Input: part model. Units: mm. Frame: model coordinates. Face numbers are marked on the shaded views. Give positions to 0.01 mm unless a question says otherwise; leave off trailing zeros. Write each loop counter-clockwise with the first axis right and the second up, starting at its lowest first coordinate (ties: lowest second). Pieces come first, ordered by that corner, then holes. Notation, with made-up numbers: (66.25, -18.5) - (122.25, -18.5) arc R16 ccw to (122.25, -9.5) - close; hole circle Ø5 at (42, 54.25). An arc over 180 degrees is marked (long way). Answer as CSV lines item,"result".
```python
from build123d import *

# Parameters (mm, degrees)
SKETCH1_R           = 7.5
BOSS_EXTRUDE1_DEPTH = 10
SKETCH2_R           = 6.5
CUT_EXTRUDE1_DEPTH  = 8.5
CAVITY1_START       = 8
CAVITY1_OUTLINE_R   = 6.6
CAVITY1_DEPTH       = 0.5


# Read off the part's stored shape, not the designer's step: Cavity1
with BuildPart() as part:
    # Sketch1 → Boss-Extrude1 (new body)
    with BuildSketch(Plane(origin=(0, 0, 0), x_dir=(1, 0, 0), z_dir=(0, 1, 0))):
        with Locations(Location((0, 0, 0), (0, 0, 270))):
            Circle(SKETCH1_R)
    extrude(amount=BOSS_EXTRUDE1_DEPTH)

    # Sketch2 → Cut-Extrude1 (cut)
    with BuildSketch(Plane(origin=(0, 10, 0), x_dir=(1, 0, 0), z_dir=(0, 1, 0))):
        with Locations(Location((0, 0, 0), (0, 0, 270))):
            Circle(SKETCH2_R)
    extrude(amount=-CUT_EXTRUDE1_DEPTH, mode=Mode.SUBTRACT)

    # Cavity1 outline → Cavity1 (cut)
    with BuildSketch(Plane(origin=(0, 0, 0), x_dir=(1, 0, 0), z_dir=(0, 1, 0)).offset(CAVITY1_START)):
        Circle(CAVITY1_OUTLINE_R)
    extrude(amount=CAVITY1_DEPTH, mode=Mode.SUBTRACT)


solid = part.part
```
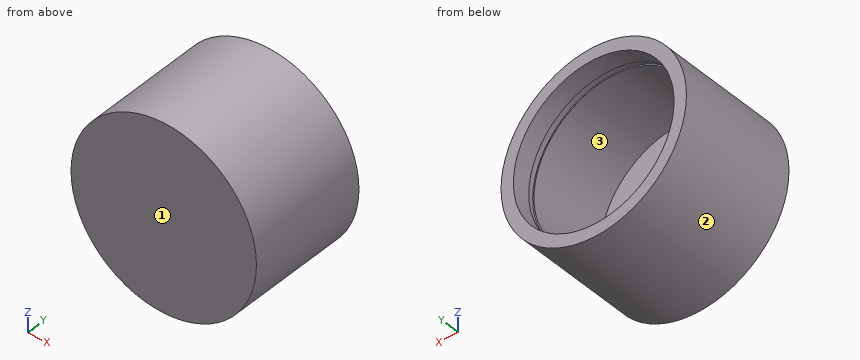
Item 1: Ray query, line 1 (X direction, y = 5.75, z = -0.25); line 2 (X direction, y = 8.35, z = 0); line 3 (Y direction, x = -4, z = 1). Return the intervals inside material, ascending. Write a range as from..to.
The answers:
line 1,"-7.5..-6.5, 6.5..7.5"
line 2,"-7.5..-6.6, 6.6..7.5"
line 3,"0..1.5"
Item 2: Cut plane B-B on y = 6. Return the cut outline in (x, z).
The answers:
outline,"circle Ø15 at (0, 0); hole circle Ø13 at (0, 0)"
Item 3: Mould query, pull axis Z, two halves, no side actions, for the marked faces 1, 2 and 3. Classes: +Z half, -Z half, draft (parallel to the pull), parting line (faces both ways), or undercut.
The answers:
face 1,"draft"
face 2,"parting line"
face 3,"undercut"
Item 4: Cut plane C-C on x = 0. Return the cut outline in (y, z).
The answers:
outline,"(0, -7.5) - (10, -7.5) - (10, -6.5) - (8.5, -6.5) - (8.5, -6.6) - (8, -6.6) - (8, -6.5) - (1.5, -6.5) - (1.5, 6.5) - (8, 6.5) - (8, 6.6) - (8.5, 6.6) - (8.5, 6.5) - (10, 6.5) - (10, 7.5) - (0, 7.5) - close"
Item 5: Cut plane A-A on z = 0. Return the cut outline in (x, y).
The answers:
outline,"(-7.5, 0) - (7.5, 0) - (7.5, 10) - (6.5, 10) - (6.5, 8.5) - (6.6, 8.5) - (6.6, 8) - (6.5, 8) - (6.5, 1.5) - (-6.5, 1.5) - (-6.5, 8) - (-6.6, 8) - (-6.6, 8.5) - (-6.5, 8.5) - (-6.5, 10) - (-7.5, 10) - close"
Item 6: Contact query for flat-ended pins moving along their axis: pin 1 (6.5 mm diameter, centred on x = -1, z = 2, fed in from +Y); pin 2 (4 mm diameter, centred on x = 4, y = 1, fed in from -Z); pin 3 (3 mm diameter, centred on x = -4, z = -2, fed in from -Y); pin 4 (3 mm diameter, centred on x = 2, y = 5, fed in from -Z). Output: stop coordinate, or through.
The answers:
pin 1,"y = 1.5"
pin 2,"z = -7.23"
pin 3,"y = 0"
pin 4,"z = -7.48"
